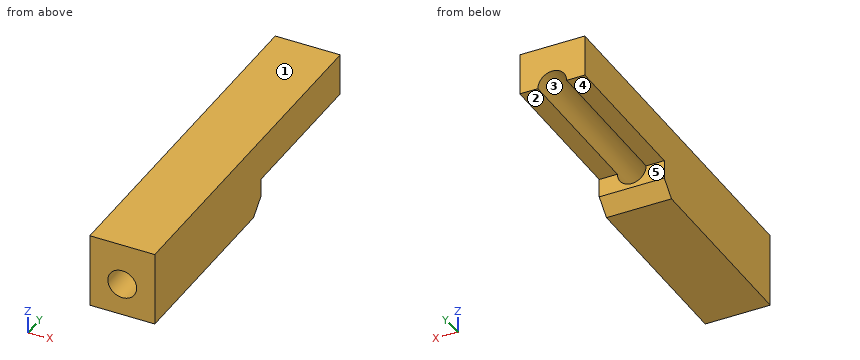
```python
from build123d import *

# Parameters (mm, degrees)
SKETCH_W       = 7
SKETCH_H       = 7
SKETCH_R       = 1.55
PAD_DEPTH      = 38.5
SKETCH001_W    = 3.5
SKETCH001_H    = 16.5
POCKET_DEPTH   = 7.001
POCKET_FACE7_W = 38.5
POCKET_FACE7_H = 7
PAD001_DEPTH   = 1
CHAMFER_SIZE   = 1.5


with BuildPart() as part:
    # Sketch → Pad (new body)
    with BuildSketch(Plane.XZ):
        Rectangle(SKETCH_W, SKETCH_H)
        Circle(SKETCH_R, mode=Mode.SUBTRACT)
    extrude(amount=PAD_DEPTH)

    # Sketch001 (on Face3 of Pad) → Pocket (cut, through all)
    with BuildSketch(Plane(origin=(3.5, 0, 0), x_dir=(0, 0, 1), z_dir=(1, 0, 0))):
        with Locations((-1.75, 8.25)):
            Rectangle(SKETCH001_W, SKETCH001_H)
    extrude(amount=-POCKET_DEPTH, mode=Mode.SUBTRACT)

    # Pocket Face7 → Pad001 (add)
    with BuildSketch(Plane(origin=(0, -19.25, 3.5), x_dir=(0, 1, 0), z_dir=(0, 0, 1))):
        Rectangle(POCKET_FACE7_W, POCKET_FACE7_H)
    extrude(amount=PAD001_DEPTH)

    # Chamfer
    chamfer_edges = [part.edges().sort_by_distance(p)[0] for p in [
        (0, -16.5, -3.5),
    ]]
    chamfer(chamfer_edges, length=CHAMFER_SIZE)


solid = part.part
```
Could you check a few things on this model? Use its own coordinates, in mm. Face numbers are marked on the shaded views. A direction names the side the tool comes from. Coordinates: 2 decimals unless noted, no trailing zeros. Loops run counter-clockwise (first coordinate to the right, second up) from the corner with the lowest first, then second, coordinate; pieces in that order, holes last.
1) Imagine slicing it at A-A (z = -0.5). List the corners of the cut face in (x, y) for me.
Reported:
outline: (-3.5, -38.5) - (-1.47, -38.5) - (-1.47, -16.5) - (-3.5, -16.5) - close; (1.47, -38.5) - (3.5, -38.5) - (3.5, -16.5) - (1.47, -16.5) - close
2) Imagine slicing it at C-C (y = -30.5). List the corners of the cut face in (x, z) for me, and give its area (3 significant figures).
Reported:
outline: (-3.5, -3.5) - (3.5, -3.5) - (3.5, 4.5) - (-3.5, 4.5) - close; hole circle Ø3.1 at (0, 0)
area: 48.5 mm2
3) Which directions (+Z, -Z, +X, -X, +Y, -Y) give clear straight access to the entire face, cutting with the end or side of a thin tool? Please do the marked faces 1 and 2.
Reported:
face 1: +Z, +X, -X, +Y, -Y
face 2: -Z, +X, -X, +Y
4) Will these pins go through, and if not, where does the flat tip stop? pin 1 Ø1.6 at (x, y) = (3, -12) entering from -Z; pin 2 Ø1 at (x, z) = (-1, -1) entering from +Y.
Reported:
pin 1: stops at z = 0
pin 2: stops at y = -16.5
5) Imagine slicing it at D-D (x = -2.75). List the corners of the cut face in (y, z) for me.
Reported:
outline: (-38.5, -3.5) - (-18, -3.5) - (-16.5, -2) - (-16.5, 0) - (0, 0) - (0, 4.5) - (-38.5, 4.5) - close
6) Imagine slicing it at B-B (x = 0). List the corners of the cut face in (y, z) for me.
Reported:
outline: (-38.5, -3.5) - (-18, -3.5) - (-16.5, -2) - (-16.5, -1.55) - (-38.5, -1.55) - close; (-38.5, 1.55) - (0, 1.55) - (0, 4.5) - (-38.5, 4.5) - close
7) Thinking about a two-plate mould opening in Z: for the marked faces 3, 4 and 5, which applies, released by +Z, released by -Z, zero draft, split by the parting line, or undercut?
Reported:
face 3: undercut
face 4: released by -Z
face 5: zero draft
8) Please list where these lines run through material, in increasing order: line 1 along X through (y, z) = (-20, 0); line 2 along Z through (x, y) = (0, -27); line 3 along Z through (x, y) = (3, -15.5).
Reported:
line 1: x = -3.5 to -1.55, 1.55 to 3.5
line 2: z = -3.5 to -1.55, 1.55 to 4.5
line 3: z = 0 to 4.5
